from build123d import *

# Parameters (mm, degrees)
F1_DEPTH = 38.1
F3_DEPTH = 19.05
F4_DEPTH = 38.1
F5_DEPTH = 25.4
F6_R     = 5.08
F7_R     = 3.175
F7_R_2   = 1.27
F8_DEPTH = 9.525
F9_DEPTH = 12.7
F10_R    = 5.08


# Not quite as in the source:
# - a feature names something its author has since deleted; it is built from what else it names


with BuildPart() as f1:
    # F0 (on Front) → F1 (new body)
    with BuildSketch(Plane.XZ):
        Polygon((19.05, -31.75), (19.05, 31.75), (-19.05, 31.75), (-19.05, 0), (-19.05, -31.75), align=None)
        with BuildLine():
            ThreePointArc((-6.35, 0), (-9.525, -3.175), (-12.7, 0))
            ThreePointArc((-12.7, 0), (-9.525, 3.175), (-6.35, 0))
        make_face(mode=Mode.SUBTRACT)
    extrude(amount=F1_DEPTH)

    # F2 (on face) → F3 (cut)
    with BuildSketch(Plane(origin=(0, 0, 0), x_dir=(-1, 0, 0), z_dir=(0, 1, 0))):
        with BuildLine():
            ThreePointArc((-8.89, 14.6707808959), (-6.2861792775, 20.956960188), (2.06e-08, 23.5607808959))
            ThreePointArc((2.06e-08, 23.5607808959), (-9.8358430758, 22.3144881592), (-19.05, 18.654383355))
            Line((-19.05, 18.654383355), (-19.05, 14.6707808959))
            Line((-19.05, 14.6707808959), (-8.89, 14.6707808959))
        make_face()
        with BuildLine():
            ThreePointArc((1.27, 14.6707808959), (0.8980256121, 15.5688065081), (0, 15.9407808959))
            Line((0, 15.9407808959), (0, 14.6707808959))
            Line((0, 14.6707808959), (1.27, 14.6707808959))
        make_face()
        with BuildLine():
            ThreePointArc((0, 13.4007808959), (0.8980256121, 13.7727552838), (1.27, 14.6707808959))
            Line((1.27, 14.6707808959), (0, 14.6707808959))
            Line((0, 14.6707808959), (0, 13.4007808959))
        make_face()
        with BuildLine():
            Line((0, 14.6707808959), (0, 15.9407808959))
            ThreePointArc((0, 15.9407808959), (-0.8980256121, 15.5688065081), (-1.27, 14.6707808959))
            Line((-1.27, 14.6707808959), (0, 14.6707808959))
        make_face()
        with BuildLine():
            Line((0, 14.6707808959), (-1.27, 14.6707808959))
            ThreePointArc((-1.27, 14.6707808959), (-0.8980256121, 13.7727552838), (0, 13.4007808959))
            Line((0, 13.4007808959), (0, 14.6707808959))
        make_face()
        with BuildLine():
            ThreePointArc((-1.6e-09, 5.7807808959), (-6.2861792853, 8.3846016118), (-8.89, 14.6707808959))
            Line((-8.89, 14.6707808959), (-19.05, 14.6707808959))
            Line((-19.05, 14.6707808959), (-19.05, -5.5759541115))
            ThreePointArc((-19.05, -5.5759541115), (-11.0891605869, 2.7261656541), (-1.6e-09, 5.7807808959))
        make_face()
        with BuildLine():
            Line((-1.27, 14.6707808959), (-8.89, 14.6707808959))
            ThreePointArc((-8.89, 14.6707808959), (-6.2861792853, 8.3846016118), (-1.6e-09, 5.7807808959))
            Line((0, 5.7807808959), (0, 6.7332808959))
            Line((0, 6.7332808959), (0, 13.4007808959))
            ThreePointArc((0, 13.4007808959), (-0.8980256121, 13.7727552838), (-1.27, 14.6707808959))
        make_face()
        with BuildLine():
            ThreePointArc((-1.6e-09, 5.7807808959), (6.2861792842, 8.3846016106), (8.89, 14.6707808959))
            Line((8.89, 14.6707808959), (1.27, 14.6707808959))
            ThreePointArc((1.27, 14.6707808959), (0.8980256121, 13.7727552838), (0, 13.4007808959))
            Line((0, 13.4007808959), (0, 6.7332808959))
            Line((0, 6.7332808959), (0, 5.7807808959))
        make_face()
        with BuildLine():
            ThreePointArc((8.89, 14.6707808959), (6.286179292, 20.9569601734), (2.06e-08, 23.5607808959))
            Line((0, 23.5607808959), (0, 22.6082808959))
            Line((0, 22.6082808959), (0, 15.9407808959))
            ThreePointArc((0, 15.9407808959), (0.8980256121, 15.5688065081), (1.27, 14.6707808959))
            Line((1.27, 14.6707808959), (8.89, 14.6707808959))
        make_face()
        with BuildLine():
            Line((0, 22.6082808959), (0, 23.5607808959))
            ThreePointArc((2.06e-08, 23.5607808959), (-6.2861792775, 20.956960188), (-8.89, 14.6707808959))
            Line((-8.89, 14.6707808959), (-1.27, 14.6707808959))
            ThreePointArc((-1.27, 14.6707808959), (-0.8980256121, 15.5688065081), (0, 15.9407808959))
            Line((0, 15.9407808959), (0, 22.6082808959))
        make_face()
    extrude(amount=-F3_DEPTH, mode=Mode.SUBTRACT)

    # F2 (on face) → F4 (cut)
    with BuildSketch(Plane(origin=(0, 0, 0), x_dir=(-1, 0, 0), z_dir=(0, 1, 0))):
        with BuildLine():
            Line((0, 14.6707808959), (0, 15.9407808959))
            ThreePointArc((0, 15.9407808959), (-0.8980256121, 15.5688065081), (-1.27, 14.6707808959))
            Line((-1.27, 14.6707808959), (0, 14.6707808959))
        make_face()
        with BuildLine():
            ThreePointArc((1.27, 14.6707808959), (0.8980256121, 15.5688065081), (0, 15.9407808959))
            Line((0, 15.9407808959), (0, 14.6707808959))
            Line((0, 14.6707808959), (1.27, 14.6707808959))
        make_face()
        with BuildLine():
            ThreePointArc((0, 13.4007808959), (0.8980256121, 13.7727552838), (1.27, 14.6707808959))
            Line((1.27, 14.6707808959), (0, 14.6707808959))
            Line((0, 14.6707808959), (0, 13.4007808959))
        make_face()
        with BuildLine():
            Line((0, 14.6707808959), (-1.27, 14.6707808959))
            ThreePointArc((-1.27, 14.6707808959), (-0.8980256121, 13.7727552838), (0, 13.4007808959))
            Line((0, 13.4007808959), (0, 14.6707808959))
        make_face()
    extrude(amount=-F4_DEPTH, mode=Mode.SUBTRACT)

    # F2 (on face) → F5 (cut)
    with BuildSketch(Plane(origin=(0, 0, 0), x_dir=(-1, 0, 0), z_dir=(0, 1, 0))):
        with BuildLine():
            ThreePointArc((12.7, -15.875), (8.9802561211, -6.8947438789), (0, -3.175))
            ThreePointArc((0, -3.175), (-8.9802561211, -6.8947438789), (-12.7, -15.875))
            ThreePointArc((-12.7, -15.875), (-8.9802561211, -24.8552561211), (0, -28.575))
            ThreePointArc((0, -28.575), (8.9802561211, -24.8552561211), (12.7, -15.875))
        make_face()
    extrude(amount=-F5_DEPTH, mode=Mode.SUBTRACT)

    # F6
    f6_edges = [f1.edges().sort_by_distance(p)[0] for p in [
        (19.05, -19.05, 31.75),
        (-19.05, -19.05, 31.75),
    ]]
    fillet(f6_edges, radius=F6_R)

    # F7 (on face) → F8 (cut)
    with BuildSketch(Plane.XZ.offset(38.1)):
        with BuildLine():
            Line((-13.97, 25.4), (-13.97, 26.67))
            Line((-13.97, 26.67), (-12.7, 26.67))
            ThreePointArc((-12.7, 26.67), (-14.8680256121, 27.5680256121), (-13.97, 25.4))
        make_face()
        with BuildLine():
            Line((-12.7, 26.67), (-13.97, 26.67))
            Line((-13.97, 26.67), (-13.97, 25.4))
            ThreePointArc((-13.97, 25.4), (-13.0719743879, 25.7719743879), (-12.7, 26.67))
        make_face()
        with BuildLine():
            Line((13.97, 26.67), (12.7, 26.67))
            ThreePointArc((12.7, 26.67), (13.0719743879, 25.7719743879), (13.97, 25.4))
            Line((13.97, 25.4), (13.97, 26.67))
        make_face()
        with BuildLine():
            ThreePointArc((15.24, 26.67), (13.97, 27.94), (12.7, 26.67))
            Line((12.7, 26.67), (13.97, 26.67))
            Line((13.97, 26.67), (13.97, 25.4))
            ThreePointArc((13.97, 25.4), (14.8680256121, 25.7719743879), (15.24, 26.67))
        make_face()
        with BuildLine():
            Line((-13.97, -25.4), (-13.97, -24.13))
            ThreePointArc((-13.97, -24.13), (-15.24, -25.4), (-13.97, -26.67))
            Line((-13.97, -26.67), (-13.97, -25.4))
        make_face()
        with BuildLine():
            ThreePointArc((-12.7, -25.4), (-13.0719743879, -24.5019743879), (-13.97, -24.13))
            Line((-13.97, -24.13), (-13.97, -25.4))
            Line((-13.97, -25.4), (-12.7, -25.4))
        make_face()
        with BuildLine():
            ThreePointArc((15.24, -25.4), (14.8680256121, -24.5019743879), (13.97, -24.13))
            Line((13.97, -24.13), (13.97, -25.4))
            Line((13.97, -25.4), (13.97, -26.67))
            ThreePointArc((13.97, -26.67), (14.8680256121, -26.2980256121), (15.24, -25.4))
        make_face()
        with BuildLine():
            Line((13.97, -25.4), (13.97, -24.13))
            ThreePointArc((13.97, -24.13), (13.0719743879, -24.5019743879), (12.7, -25.4))
            Line((12.7, -25.4), (13.97, -25.4))
        make_face()
        with BuildLine():
            Line((13.97, -25.4), (12.7, -25.4))
            ThreePointArc((12.7, -25.4), (13.0719743879, -26.2980256121), (13.97, -26.67))
            Line((13.97, -26.67), (13.97, -25.4))
        make_face()
        with BuildLine():
            Line((-12.7, -25.4), (-13.97, -25.4))
            Line((-13.97, -25.4), (-13.97, -26.67))
            ThreePointArc((-13.97, -26.67), (-13.0719743879, -26.2980256121), (-12.7, -25.4))
        make_face()
        with Locations((0, 14.6707808959)):
            Circle(F7_R)
        with Locations((0, 14.6707808959)):
            Circle(F7_R_2, mode=Mode.SUBTRACT)
    extrude(amount=-F8_DEPTH, mode=Mode.SUBTRACT)

    # F7 (on face) → F9 (cut)
    with BuildSketch(Plane.XZ.offset(38.1)):
        with BuildLine():
            Line((-12.7, 26.67), (-13.97, 26.67))
            Line((-13.97, 26.67), (-13.97, 25.4))
            ThreePointArc((-13.97, 25.4), (-13.0719743879, 25.7719743879), (-12.7, 26.67))
        make_face()
        with BuildLine():
            Line((-13.97, 25.4), (-13.97, 26.67))
            Line((-13.97, 26.67), (-12.7, 26.67))
            ThreePointArc((-12.7, 26.67), (-14.8680256121, 27.5680256121), (-13.97, 25.4))
        make_face()
        with BuildLine():
            Line((13.97, 26.67), (12.7, 26.67))
            ThreePointArc((12.7, 26.67), (13.0719743879, 25.7719743879), (13.97, 25.4))
            Line((13.97, 25.4), (13.97, 26.67))
        make_face()
        with BuildLine():
            ThreePointArc((15.24, 26.67), (13.97, 27.94), (12.7, 26.67))
            Line((12.7, 26.67), (13.97, 26.67))
            Line((13.97, 26.67), (13.97, 25.4))
            ThreePointArc((13.97, 25.4), (14.8680256121, 25.7719743879), (15.24, 26.67))
        make_face()
        with BuildLine():
            ThreePointArc((15.24, -25.4), (14.8680256121, -24.5019743879), (13.97, -24.13))
            Line((13.97, -24.13), (13.97, -25.4))
            Line((13.97, -25.4), (13.97, -26.67))
            ThreePointArc((13.97, -26.67), (14.8680256121, -26.2980256121), (15.24, -25.4))
        make_face()
        with BuildLine():
            Line((13.97, -25.4), (13.97, -24.13))
            ThreePointArc((13.97, -24.13), (13.0719743879, -24.5019743879), (12.7, -25.4))
            Line((12.7, -25.4), (13.97, -25.4))
        make_face()
        with BuildLine():
            Line((13.97, -25.4), (12.7, -25.4))
            ThreePointArc((12.7, -25.4), (13.0719743879, -26.2980256121), (13.97, -26.67))
            Line((13.97, -26.67), (13.97, -25.4))
        make_face()
        with BuildLine():
            Line((-12.7, -25.4), (-13.97, -25.4))
            Line((-13.97, -25.4), (-13.97, -26.67))
            ThreePointArc((-13.97, -26.67), (-13.0719743879, -26.2980256121), (-12.7, -25.4))
        make_face()
        with BuildLine():
            ThreePointArc((-12.7, -25.4), (-13.0719743879, -24.5019743879), (-13.97, -24.13))
            Line((-13.97, -24.13), (-13.97, -25.4))
            Line((-13.97, -25.4), (-12.7, -25.4))
        make_face()
        with BuildLine():
            Line((-13.97, -25.4), (-13.97, -24.13))
            ThreePointArc((-13.97, -24.13), (-15.24, -25.4), (-13.97, -26.67))
            Line((-13.97, -26.67), (-13.97, -25.4))
        make_face()
    extrude(amount=-F9_DEPTH, mode=Mode.SUBTRACT)

    # F10
    f10_edges = [f1.edges().sort_by_distance(p)[0] for p in [
        (19.05, -19.05, -31.75),
        (-19.05, -19.05, -31.75),
    ]]
    fillet(f10_edges, radius=F10_R)


solid = f1.part
Can you work these out from the model? Positions are in its coordinate system, mm. A direction names the side the tool comes from. Give positions to 0.01 mm unless a question says otherwise; leave off trailing zeros. Order: outer loops, then holes, each group sorted by start corner. A loop starts at its lowest first (then second) coordinate and runs counter-clockwise, first axis right, second up. Notation, with made-up numbers: M 89.5,-8 L 98.5,-8 A19 ccw 98.5,21 Z; hole C 7.5,-8 d5. An arc over 180 degrees is marked long. Use a Markdown table: item, result. Add a question column.
Item 1: Will these pins go through, and if not, where does the flat tip stop? pin 1 (2 mm diameter, centred on x = 13.97, z = 26.67, fed in from +Y); pin 2 (4 mm diameter, centred on x = -9.525, z = 0, fed in from +Y); pin 3 (4 mm diameter, centred on y = -16, z = 4, fed in from +X); pin 4 (5 mm diameter, centred on x = 0, z = 14.67, fed in from -Y) (3 decimals).
Item 2: Suppose I cut it at D-D (z = -17.5). List the corners of the cut face in (x, y) for me, then the cut area to 3 significant figures.
Item 3: For faces 1 (the cylindrical face through (17.601, -19.317, 30.222)), 2 (the flat face through (-14, -25.4, 27)), 3 (the cylindrical face through (9.7, -9.39, 22.35)), which set-ups out of +Z, -Z, +X, -X, +Y, -Y let a thin tool reach every point of the face, with its end or its side?
Item 4: Suppose I cut it at A-A (z = 2.5). List the corners of the cut face in (x, y) for me, then the cut area to 3 significant figures.
Item 5: Suppose I cut it at B-B (y = -32). List the corners of the cut face in (x, z) for me (3 decimals), then the cut area to 3 significant figures.
Item 6: We'd pull the mould along X, two halves only. Please class faces 4 (the flat face through (0, -38.1, 0)), 5 (the cylindrical face through (-0.69, -33.4, 11.57)), 6 (the flat face through (-19.05, -19, 0)), 7 (the flat face through (19.05, -23, 0)): +X half, -X half, draft (parallel to the pull), parting line (faces both ways), or undercut.
Item 7: Suppose I cut it at C-C (y = -18). List the corners of the cut face in (x, z) for me (3 decimals).
Item 8: If I drill on L1, parallel to Z at x = -13.97, y = -30.75; L2, parallel to X at y = -32.5, z = -25.4; L3, parallel to Z at x = 13, y = -34, over which ranges is the centre line in solid material (lowest first)? Write a range as [from, to].
Answer sheet:
| question | item | result |
|---|---|---|
| 1 | pin 1 | stops at y = 0 |
| 1 | pin 2 | passes through |
| 1 | pin 3 | stops at x = 12.23 |
| 1 | pin 4 | stops at y = -28.575 |
| 2 | outline | M -19.05,-38.1 L 19.05,-38.1 L 19.05,0 L 12.6,0 L 12.6,-25.4 L -12.6,-25.4 L -12.6,0 L -19.05,0 Z |
| 2 | area | 812 mm² |
| 3 | face 1 | +Z, +X, +Y, -Y |
| 3 | face 2 | -Y |
| 3 | face 3 | +Y |
| 4 | outline | M -19.05,-38.1 L -11.48,-38.1 L -11.48,0 L -19.05,0 Z; M -7.57,-38.1 L 19.05,-38.1 L 19.05,-19.05 L 11.46,-19.05 L 11.46,0 L -7.57,0 Z |
| 4 | area | 1,160 mm² |
| 5 | outline | M -19.05,-26.67 A5.08 ccw -13.97,-31.75 L 13.97,-31.75 A5.08 ccw 19.05,-26.67 L 19.05,26.67 A5.08 ccw 13.97,31.75 L -13.97,31.75 A5.08 ccw -19.05,26.67 Z; hole C -13.97,-25.4 d2.54; hole C -13.97,26.67 d2.54; hole C -9.525,0 d6.35; hole C 0,14.671 d6.35; hole C 13.97,-25.4 d2.54; hole C 13.97,26.67 d2.54 |
| 5 | area | 2,310 mm² |
| 6 | face 4 | draft |
| 6 | face 5 | undercut |
| 6 | face 6 | -X half |
| 6 | face 7 | +X half |
| 7 | outline | M -19.05,-26.67 A5.08 ccw -13.97,-31.75 L 13.97,-31.75 A5.08 ccw 19.05,-26.67 L 19.05,-5.576 A21.656 ccw 0,5.781 A8.89 cw 0,23.561 A39.436 cw 19.05,18.654 L 19.05,26.67 A5.08 ccw 13.97,31.75 L -13.97,31.75 A5.08 ccw -19.05,26.67 Z; hole C 0,-15.875 d25.4; hole C -9.525,0 d6.35 |
| 8 | L1 | z = [-31.75, -26.67], [-24.13, 25.4], [27.94, 31.75] |
| 8 | L2 | x = [-19.05, -15.24], [-12.7, 12.7], [15.24, 19.05] |
| 8 | L3 | z = [-31.75, -26.22], [-24.58, 25.85], [27.49, 31.75] |
